from build123d import *

# Parameters (mm, degrees)
SKETCH1_W           = 20
SKETCH1_H           = 40
SKETCH1_R           = 2
BOSS_EXTRUDE1_DEPTH = 1.5
SKETCH2_W           = 20
SKETCH2_H           = 1.5
BOSS_EXTRUDE2_DEPTH = 38.5
SKETCH3_R           = 2
CUT_EXTRUDE1_DEPTH  = 1.5


with BuildPart() as part:
    # Sketch1 → Boss-Extrude1 (new body)
    with BuildSketch(Plane(origin=(0, 0, 0), x_dir=(1, 0, 0), z_dir=(0, 1, 0))):
        Rectangle(SKETCH1_W, SKETCH1_H)
        with Locations((0, -5)):
            Circle(SKETCH1_R, mode=Mode.SUBTRACT)
    extrude(amount=BOSS_EXTRUDE1_DEPTH)

    # Sketch2 → Boss-Extrude2 (add)
    with BuildSketch(Plane(origin=(0, 1.5, 0), x_dir=(1, 0, 0), z_dir=(0, 1, 0))):
        with Locations((0, 19.25)):
            Rectangle(SKETCH2_W, SKETCH2_H)
    extrude(amount=BOSS_EXTRUDE2_DEPTH)

    # Sketch3 → Cut-Extrude1 (cut)
    with BuildSketch(Plane(origin=(0, 0, -20), x_dir=(-1, 0, 0), z_dir=(0, 0, -1))):
        with Locations((0, 25)):
            Circle(SKETCH3_R)
    extrude(amount=-CUT_EXTRUDE1_DEPTH, mode=Mode.SUBTRACT)


solid = part.part
Source: CAD feature listing. Evaluate the final solid. Frame: model axes, mm. A direction names the side the tool comes from. Coordinates: 2 decimals unless noted, no trailing zeros. Loops run counter-clockwise (first coordinate to the right, second up) from the corner with the lowest first, then second, coordinate; pieces in that order, holes last. Notation, with made-up numbers: (43.5, 26) - (84.5, 26) arc R11 cw to (84.5, 45) - close; hole circle Ø7 at (79.25, -9.75). An arc over 180 degrees is marked (long way). One line per item, written item: value. Start each with the question number.
1. Section C-C (y = 25). Return the cut outline in (x, z).
2. Mould query, pull axis X, two halves, no side actions, for faces 3 (the cylindrical face through (0, 23, -19)), 4 (the flat face through (0, 20, -18.5)), 5 (the flat face through (10, 11, -19)). Classes: pulls with the +X half, pulls with the -X half, needs draft (parallel to the pull), parting line crosses it, or undercut.
3. Section D-D (z = -11.5). Return the cut outline in (x, y), and give its area (3 significant figures).
4. Section A-A (z = 5). Return the cut outline in (x, y), and give its area (3 significant figures).
5. Contact query for a flat-ended pin moving along its axis: P1, Ø6, axis at x = -2.5, y = 18, coming from the +Z side. Output: stop coordinate, or through.
6. Ray query, L1, parallel to Y at x = 0, z = -19.05; L2, parallel to Z at x = 0, y = 0.6; L3, parallel to Y at x = -8.5, z = 10. Return the intervals inside material, ascending.
7. Set-up query: faces 1 (the flat face through (0, 0, 0)), 2 (the flat face through (0, 1.5, 0)). Return all of +Z, -Z, +X, -X, +Y, -Y with unobstructed straight access to the full face (end or side cutting, diameter ignored); none if empty.
8. Section B-B (x = 0). Return the cut outline in (y, z).
Verdict:
1. outline: (-10, -20) - (-2, -20) - (-2, -18.5) - (-10, -18.5) - close; (2, -20) - (10, -20) - (10, -18.5) - (2, -18.5) - close
2. face 3: undercut
2. face 4: needs draft
2. face 5: pulls with the +X half
3. outline: (-10, 0) - (10, 0) - (10, 1.5) - (-10, 1.5) - close
3. area: 30.0 mm2
4. outline: (-10, 0) - (-2, 0) - (-2, 1.5) - (-10, 1.5) - close; (2, 0) - (10, 0) - (10, 1.5) - (2, 1.5) - close
4. area: 24.0 mm2
5. P1: stops at z = -18.5
6. L1: y = 0 to 23, 27 to 40
6. L2: z = -20 to 3, 7 to 20
6. L3: y = 0 to 1.5
7. face 1: +Z, -Z, +X, -X, -Y
7. face 2: +Z, +X, -X, +Y
8. outline: (0, -20) - (23, -20) - (23, -18.5) - (1.5, -18.5) - (1.5, 3) - (0, 3) - close; (0, 7) - (1.5, 7) - (1.5, 20) - (0, 20) - close; (27, -20) - (40, -20) - (40, -18.5) - (27, -18.5) - close
